Geometry check sheet. Reference: the model listing, model coordinates, mm. Face numbers are marked on the shaded views. A direction names the side the tool comes from. Round coordinates to 2 decimals unless told otherwise and drop trailing zeros. Write each loop counter-clockwise with the first axis right and the second up, starting at its lowest first coordinate (ties: lowest second). Pieces come first, ordered by that corner, then holes.
Item 1: Cross-section at C-C (z = 6). Enter the section's corners in (x, y), then the cut area to 3 significant figures.
Item 2: Cross-section at D-D (z = 12.5). Enter the section's corners in (x, y), then the cut area to 3 significant figures.
Item 3: Cross-section at A-A (x = 0). Enter the section's corners in (y, z).
Item 4: Depth check by flat-ended pin: P1, Ø4, axis at y = 3, z = 15.5, coming from the +X side; P2, Ø12, axis at y = 6.5, z = 8.5, coming from the -X side; P3, Ø4, axis at x = -2.5, z = 12.5, coming from the -Y side. Enter the tip coordinate at first touch or a pass-through.
Item 5: Access from +Z, -Z, +X, -X, +Y, -Y to the whole of each face (thin tool, end or side, straight path). Record for the marked faces 1 and 2.
Item 6: Scan lines: probe 1 along Z at (x, y) = (10.75, 5.5); probe 2 along Y at (x, z) = (-7.75, 9.25); probe 3 along Y at (x, z) = (2.5, 15.5). Record each from-to range of solid material in increasing order.
from build123d import *

# Parameters (mm, degrees)
SKETCH_1_R      = 11
EXTRUDE_1_DEPTH = 10
SKETCH_2_R      = 13
EXTRUDE_2_DEPTH = 10
EXTRUDE_2_TAPER = 3
FILLET_1_R      = 1
SKETCH_3_R      = 10.5
EXTRUDE_3_DEPTH = 2
FILLET_2_R      = 0.5


with BuildPart() as part:
    # 草图1 → 凸台-拉伸1 (new body)
    with BuildSketch(Plane.XY):
        Circle(SKETCH_1_R)
    extrude(amount=EXTRUDE_1_DEPTH)

    # 草图2 → 凸台-拉伸2 (add)
    with BuildSketch(Plane.XY.offset(10)):
        Circle(SKETCH_2_R)
    extrude(amount=EXTRUDE_2_DEPTH, taper=EXTRUDE_2_TAPER)

    # 圆角1
    fillet_1_edges = [part.edges().sort_by_distance(p)[0] for p in [
        (-12.475922207, 0, 20),
    ]]
    fillet(fillet_1_edges, radius=FILLET_1_R)

    # 草图3 → 凸台-拉伸3 (add)
    with BuildSketch(Plane.XY.offset(20)):
        Circle(SKETCH_3_R)
    extrude(amount=EXTRUDE_3_DEPTH)

    # 圆角2
    fillet_2_edges = [part.edges().sort_by_distance(p)[0] for p in [
        (-10.5, 0, 22),
    ]]
    fillet(fillet_2_edges, radius=FILLET_2_R)


solid = part.part
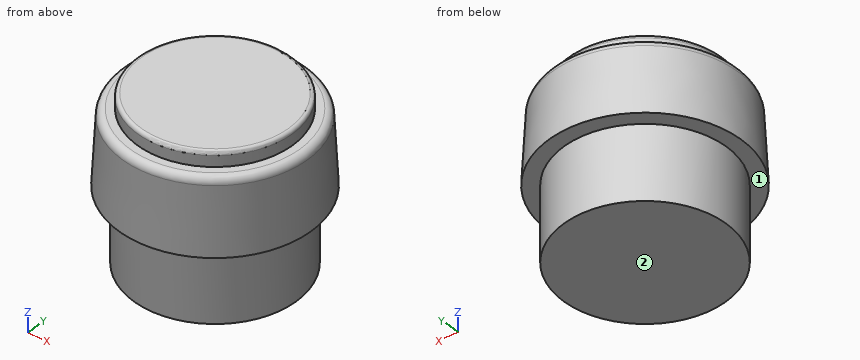
Resolved:
1. outline: circle Ø22 at (0, 0)
1. area: 380 mm2
2. outline: circle Ø25.74 at (0, 0)
2. area: 520 mm2
3. outline: (-13, 10) - (-11, 10) - (-11, 0) - (11, 0) - (11, 10) - (13, 10) - (12.53, 19.05) arc R1 ccw to (11.53, 20) - (10.5, 20) - (10.5, 21.5) arc R0.5 ccw to (10, 22) - (-10, 22) arc R0.5 ccw to (-10.5, 21.5) - (-10.5, 20) - (-11.53, 20) arc R1 ccw to (-12.53, 19.05) - close
4. P1: stops at x = 12.7
4. P2: stops at x = -12.98
4. P3: stops at y = -12.9
5. face 1: -Z
5. face 2: -Z, +X, -X, +Y, -Y
6. probe 1: z = 10 to 19.84
6. probe 2: y = -7.81 to 7.81
6. probe 3: y = -12.46 to 12.46
